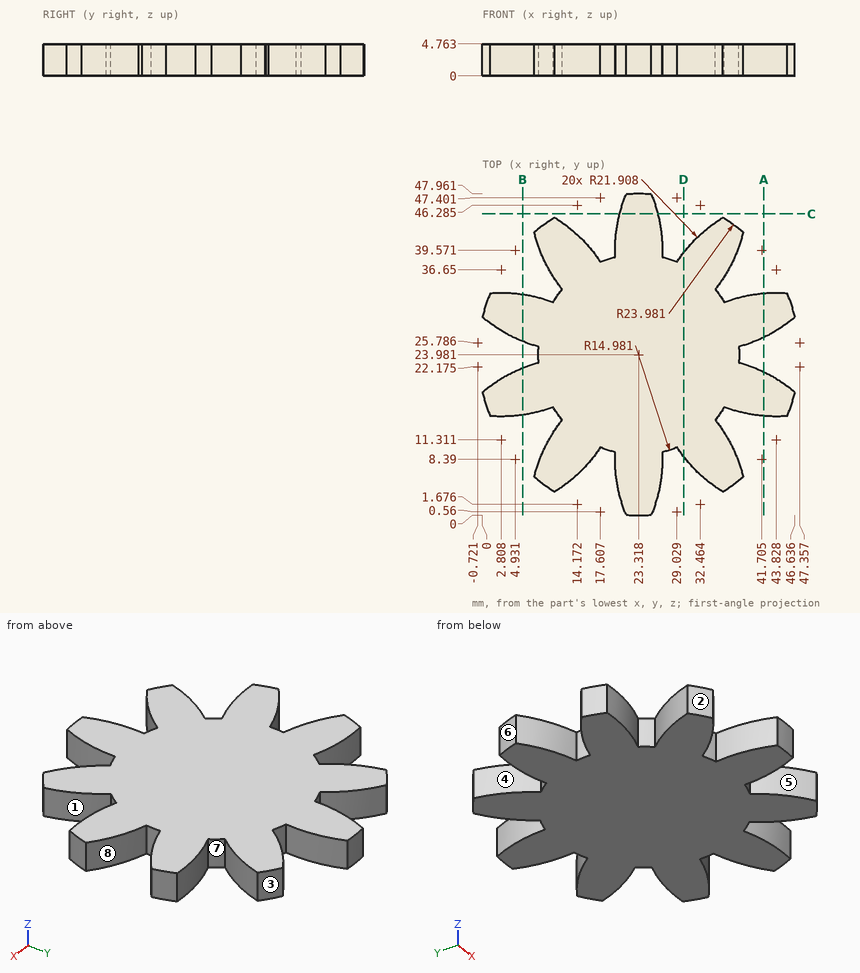
Verification items for this drawing (mm, ordinates from the low corner). A direction names the side the tool comes from. Coordinates: 2 decimals unless noted, no trailing zeros. Loops run counter-clockwise (first coordinate to the right, second up) from the corner with the lowest first, then second, coordinate; pieces in that order, holes last. Notation, with made-up numbers: (89.25, 65.5) - (121.25, 65.5) arc R19 ccw to (121.25, 100.5) - close; hole circle Ø2 at (3, 13). An arc over 180 degrees is marked (long way). One line per item, written item: value. Start each with the question number.
(1) Mould release check, pull along Y, two halves, no side actions. Record for the marked faces 1, 2 and 3: released by +Y, released by -Y, zero draft, split by the parting line, or undercut.
(2) Cross-section at D-D on x = 30. Enter the section's corners in (y, z).
(3) Cross-section at A-A on x = 42. Enter the section's corners in (y, z).
(4) Depth check by flat-ended pin: P1, Ø8, axis at x = 16, y = 33, coming from the -Z side; P2, Ø4, axis at x = 41.5, y = 10, coming from the +Z side. Enter the tip coordinate at first touch or a pass-through.
(5) Cross-section at C-C on y = 45. Enter the section's corners in (x, z) (1 decimal).
(6) Material ranges on line 1 (Y direction, x = 36, z = 3.8) (1 decimal); line 2 (X direction, y = 7, z = 1.05) (1 decimal); line 3 (X direction, y = 39, z = 2.3) (1 decimal), recorded low to high. Write a range as [from, to].
(7) Tool access check on the marked faces 4, 5, 6, 7 and 8. Record the directions out of +Z, -Z, +X, -X, +Y, -Y that give a thin tool (end or side, any length) a straight path to the whole face; none if there is none.
(8) Cross-section at B-B on x = 6. Enter the section's corners in (y, z) (1 decimal).
Results below:
1. face 1: undercut
1. face 2: released by -Y
1. face 3: released by +Y
2. outline: (8.81, 0) - (39.15, 0) - (39.15, 4.76) - (8.81, 4.76) - close
3. outline: (14.82, 0) - (21.4, 0) - (21.4, 4.76) - (14.82, 4.76) - close; (26.56, 0) - (33.14, 0) - (33.14, 4.76) - (26.56, 4.76) - close
4. P1: stops at z = 0
4. P2: passes through
5. outline: (20.5, 0) - (26.2, 0) - (26.2, 4.8) - (20.5, 4.8) - close
6. line 1: y = [3.6, 12.5], [16, 32], [35.5, 44.3]
6. line 2: x = [8.1, 15.1], [19.8, 26.8], [31.6, 38.5]
6. line 3: x = [8.8, 16.8], [19.8, 26.8], [29.9, 37.8]
7. face 4: +Z, -Z, -X
7. face 5: +Z, -Z, -Y
7. face 6: +Z, -Z, -X, +Y
7. face 7: +Z, -Z
7. face 8: +Z, -Z, +X
8. outline: (15, 0) - (22, 0) - (22, 4.8) - (15, 4.8) - close; (26, 0) - (33, 0) - (33, 4.8) - (26, 4.8) - close
